```python
from build123d import *

# Parameters (mm, degrees)
MODEL_W             = 60
MODEL_H             = 50
MODEL_R             = 2.57574226
MODEL_R_2           = 1
MODEL_W_2           = 1.778
MODEL_H_2           = 3.556
MODEL_W_3           = 3.45000072
MODEL_H_3           = 3.45000072
BOSS_EXTRUDE1_DEPTH = 1.6


with BuildPart() as part:
    # Model → Boss-Extrude1 (new body)
    with BuildSketch(Plane.XY):
        with Locations((112.002348606, 75.004629004)):
            Rectangle(MODEL_W, MODEL_H)
        with Locations((112.002348606, 73.693071842)):
            Circle(MODEL_R, mode=Mode.SUBTRACT)
        with Locations((87.002348606, 95.004629004)):
            Circle(MODEL_R_2, mode=Mode.SUBTRACT)
        with Locations(Location((137.002348606, 95.004629004, 0), (0, 0, 180))):
            Circle(MODEL_R_2, mode=Mode.SUBTRACT)
        with Locations((137.002348606, 55.004629004)):
            Circle(MODEL_R_2, mode=Mode.SUBTRACT)
        with Locations(Location((87.002348606, 55.004629004, 0), (0, 0, 180))):
            Circle(MODEL_R_2, mode=Mode.SUBTRACT)
        with Locations((121.3499986, 79.75000052)):
            Rectangle(MODEL_W_2, MODEL_H_2, mode=Mode.SUBTRACT)
        with Locations((102.75000024, 79.7749992)):
            Rectangle(MODEL_W_2, MODEL_H_2, mode=Mode.SUBTRACT)
        with Locations((111.99999952, 80.44520106)):
            Rectangle(MODEL_W_3, MODEL_H_3, mode=Mode.SUBTRACT)
        with Locations((111.99999952, 67.25000012)):
            Rectangle(MODEL_W_3, MODEL_H_3, mode=Mode.SUBTRACT)
    extrude(amount=BOSS_EXTRUDE1_DEPTH)


solid = part.part
```
Source: CAD feature listing. Evaluate the final solid. Frame: model axes, mm. A direction names the side the tool comes from. Coordinates: 2 decimals unless noted, no trailing zeros. Answer as CSV lines item,"result".
1. Ray query, line 1 (X direction, y = 55, z = 0.6); line 2 (X direction, y = 79.5, z = 0.2) (3 decimals); line 3 (Y direction, x = 103, z = 0.1). Return the intervals inside material, ascending.
Established:
line 1,"x = 82 to 86, 88 to 136, 138 to 142"
line 2,"x = 82.002 to 101.861, 103.639 to 110.275, 113.725 to 120.461, 122.239 to 142.002"
line 3,"y = 50 to 78, 81.55 to 100"
2. Contact query for flat-ended pins moving along their axis: pin 1 (4.5 mm diameter, centred on x = 112, y = 73.69, fed in from -Z); pin 2 (2.5 mm diameter, centred on x = 137, y = 55, fed in from -Z). Output: stop coordinate, or through.
Established:
pin 1,"passes through"
pin 2,"stops at z = 0"
3. Reachability of faces 1 (the flat face through (103, 77.997, 1)), 2 (the flat face through (142.002, 75, 1)) from +Z, -Z, +X, -X, +Y, -Y: full face, straight path, thin tool, end or side. Return the list, or none.
Established:
face 1,"+Z, -Z"
face 2,"+Z, -Z, +X, +Y, -Y"
4. Mould query, pull axis Y, two halves, no side actions, for faces 3 (the flat face through (112, 70, 1.6)), 4 (the flat face through (112, 100.005, 1)), 5 (the flat face through (121, 81.528, 1)), 6 (the flat face through (103, 81.553, 1)). Classes: released by +Y, released by -Y, zero draft, split by the parting line, or undercut.
Established:
face 3,"zero draft"
face 4,"released by +Y"
face 5,"undercut"
face 6,"undercut"
5. Section A-A (z = 1.35). Count the separate pieces of the cut face and the enclosed holes in it, then the cut area to 3 significant figures.
Established:
separate pieces,"1"
enclosed holes,"9"
area,"2,930 mm2"
